```python
from build123d import *

# Parameters (mm, degrees)
SKETCH2_W           = 25
SKETCH2_H           = 25
BOSS_EXTRUDE2_DEPTH = 3
SKETCH3_R           = 1.5
BOSS_EXTRUDE3_DEPTH = 3
SKETCH4_W           = 15
SKETCH4_H           = 25
BOSS_EXTRUDE4_DEPTH = 3


with BuildPart() as part:
    # Sketch2 → Boss-Extrude2 (new body)
    with BuildSketch(Plane.XY):
        Rectangle(SKETCH2_W, SKETCH2_H)
    extrude(amount=BOSS_EXTRUDE2_DEPTH)

    # Sketch3 → Boss-Extrude3 (add)
    with BuildSketch(Plane.XY.offset(3)):
        Circle(SKETCH3_R)
    extrude(amount=BOSS_EXTRUDE3_DEPTH)

    # Sketch4 → Boss-Extrude4 (add)
    with BuildSketch(Plane.XY.offset(6)):
        Rectangle(SKETCH4_W, SKETCH4_H)
    extrude(amount=BOSS_EXTRUDE4_DEPTH)


solid = part.part
```
Read the model definition and answer for the solid it produces. Units are mm, in the model's axes. A direction names the side the tool comes from. Give positions to 0.01 mm unless a question says otherwise; leave off trailing zeros. Order: outer loops, then holes, each group sorted by start corner. A loop starts at its lowest first (then second) coordinate and runs counter-clockwise, first axis right, second up. Notation, with made-up numbers: (-40, 83) -> (-8, 83) arc R15 ccw to (-8, 105) -> close; hole circle Ø10 at (40, 70). An arc over 180 degrees is marked (long way). One line per item, written item: value. Start each with the question number.
(1) A tool of negligible diameter and unlimited length cuts with its end or side. For faces 4 (the flat face through (0, 12.5, 7)), 5 (the flat face through (0, -12.5, 1)), 6 (the cylindrical face through (-1.5, 0.07, 4.48)), 7 (the flat face through (-7.5, 0, 7)), 8 (the flat face through (7.5, 0, 7)), from which of +Z, -Z, +X, -X, +Y, -Y can it reach the whole face along a straight path? Write none if from no direction.
(2) Straight lines are drawn through the part: L1, parallel to Z at x = 2, y = 1; L2, parallel to X at y = -10.5, z = 6.5; L3, parallel to Z at x = -9.5, y = 4. For each, find the intervals that lie inside material, in ascending order.
(3) The part is cut by section B-B (x = 0). Determine the outline of the cut face in (y, z).
(4) The part is cut by section C-C (x = 6.75). Determine the outline of the cut face in (y, z).
(5) The part is cut by section D-D (y = 0). Determine the outline of the cut face in (x, z), and give its area (3 significant figures).
(6) For a pull along Z with two mould halves and no side action, classify faces 1 (the flat face through (0, 0, 0)), 2 (the flat face through (-2, 0, 6)), 3 (the flat face through (0, 0, 9)) as released by +Z, released by -Z, zero draft, split by the parting line, or undercut.
(7) The part is cut by section A-A (y = 6). Determine the outline of the cut face in (x, z).
(8) Flat-ended cylindrical pins translate along their axes: P1, Ø1.5, axis at y = 0, z = 7, coming from the -X side; P2, Ø3.5, axis at y = -2, z = 7.5, coming from the +X side. Find the tip coordinate at first contact, or state that the pin passes through.
Taken from the geometry:
1. face 4: +Z, -Z, +X, -X, +Y
1. face 5: +Z, -Z, +X, -X, -Y
1. face 6: none
1. face 7: +Z, -X, +Y, -Y
1. face 8: +Z, +X, +Y, -Y
2. L1: 0 to 3, 6 to 9
2. L2: -7.5 to 7.5
2. L3: 0 to 3
3. outline: (-12.5, 0) -> (12.5, 0) -> (12.5, 3) -> (1.5, 3) -> (1.5, 6) -> (12.5, 6) -> (12.5, 9) -> (-12.5, 9) -> (-12.5, 6) -> (-1.5, 6) -> (-1.5, 3) -> (-12.5, 3) -> close
4. outline: (-12.5, 0) -> (12.5, 0) -> (12.5, 3) -> (-12.5, 3) -> close; (-12.5, 6) -> (12.5, 6) -> (12.5, 9) -> (-12.5, 9) -> close
5. outline: (-12.5, 0) -> (12.5, 0) -> (12.5, 3) -> (1.5, 3) -> (1.5, 6) -> (7.5, 6) -> (7.5, 9) -> (-7.5, 9) -> (-7.5, 6) -> (-1.5, 6) -> (-1.5, 3) -> (-12.5, 3) -> close
5. area: 129 mm^2
6. face 1: released by -Z
6. face 2: undercut
6. face 3: released by +Z
7. outline: (-12.5, 0) -> (12.5, 0) -> (12.5, 3) -> (-12.5, 3) -> close; (-7.5, 6) -> (7.5, 6) -> (7.5, 9) -> (-7.5, 9) -> close
8. P1: x = -7.5
8. P2: x = 7.5
